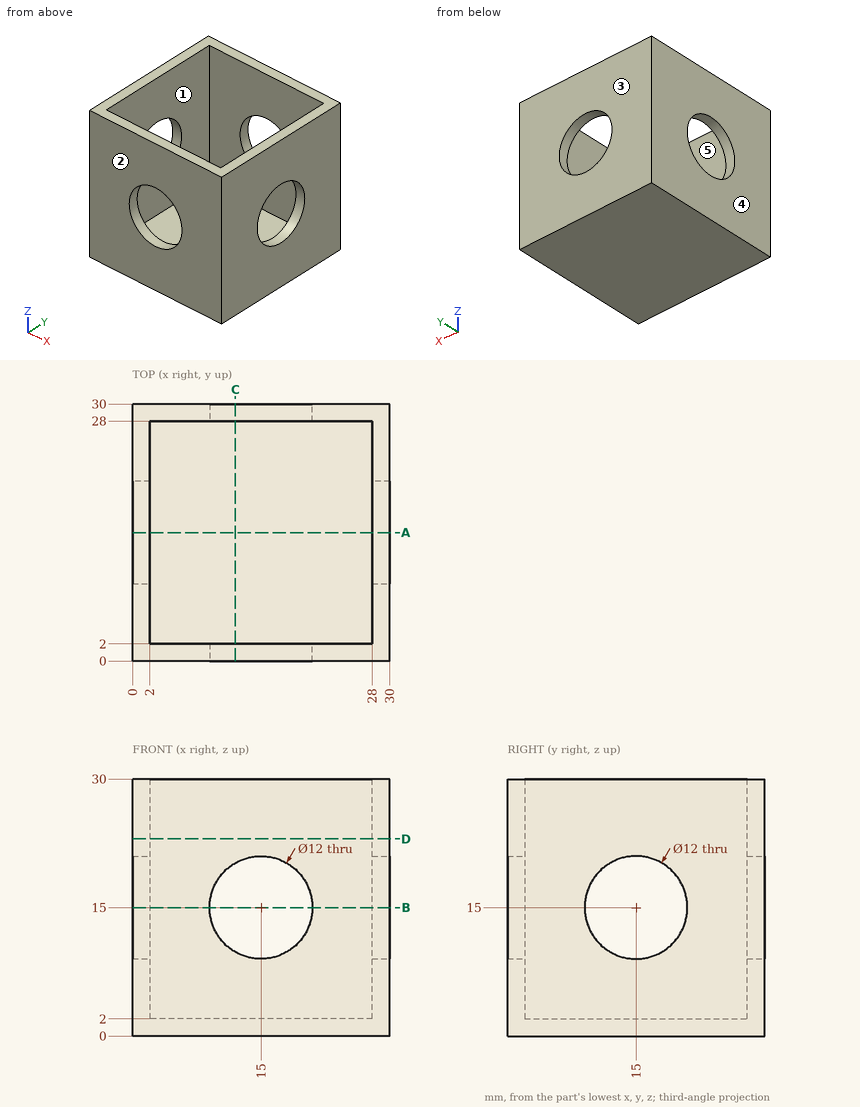
Geometry: see drawing. Coordinates: mm, zero at the bounding-box minimum. A direction names the side the tool comes from. Coordinates: 2 decimals unless noted, no trailing zeros. Order: outer loops, then holes, each group sorted by start corner. A loop starts at its lowest first (then second) coordinate and runs counter-clockwise, first axis right, second up. Notation, with made-up numbers: M 9,21 L 35,21 A18 cw 35,36 Z; hole C 56.5,31 d10. An arc over 180 degrees is marked long. Answer in a Markdown table with one row per item. Add a question column.
Q1. Section query C-C on x = 12. Return the cut outline in (y, z).
Q2. Mould query, pull axis Y, two halves, no side actions, for the marked faces 3, 4 and 5. Classes: released by +Y, released by -Y, zero draft, split by the parting line, or undercut.
Q3. Reachability of the marked faces 1 and 2 from +Z, -Z, +X, -X, +Y, -Y: full face, straight path, thin tool, end or side. Return the list, or none.
Q4. Section query B-B on z = 15. Return the cut outline in (x, y), and give its area (3 significant figures).
Q5. Contact query for a flat-ended pin moving along its axis: P1, Ø9.5, axis at x = 15, z = 15, coming from the +Y side. Output: stop coordinate, or through.
Q6. Section query A-A on y = 15. Return the cut outline in (x, z).
Q7. Section query D-D on z = 23. Return the cut outline in (x, y).
Q8. Line query: L1, parallel to Y at x = 17.5, z = 4.75; L2, parallel to Z at x = 15, y = 28.55. Output: solid intervals per line, ascending.
Completed:
| question | item | result |
|---|---|---|
| 1 | outline | M 0,0 L 30,0 L 30,9.8 L 28,9.8 L 28,2 L 2,2 L 2,9.8 L 0,9.8 Z; M 0,20.2 L 2,20.2 L 2,30 L 0,30 Z; M 28,20.2 L 30,20.2 L 30,30 L 28,30 Z |
| 2 | face 3 | released by +Y |
| 2 | face 4 | zero draft |
| 2 | face 5 | undercut |
| 3 | face 1 | +Z |
| 3 | face 2 | +Z, -Z, +X, -X, -Y |
| 4 | outline | M 0,0 L 9,0 L 9,2 L 2,2 L 2,9 L 0,9 Z; M 0,21 L 2,21 L 2,28 L 9,28 L 9,30 L 0,30 Z; M 21,0 L 30,0 L 30,9 L 28,9 L 28,2 L 21,2 Z; M 21,28 L 28,28 L 28,21 L 30,21 L 30,30 L 21,30 Z |
| 4 | area | 128 mm2 |
| 5 | P1 | passes through |
| 6 | outline | M 0,0 L 30,0 L 30,9 L 28,9 L 28,2 L 2,2 L 2,9 L 0,9 Z; M 0,21 L 2,21 L 2,30 L 0,30 Z; M 28,21 L 30,21 L 30,30 L 28,30 Z |
| 7 | outline | M 0,0 L 30,0 L 30,30 L 0,30 Z; hole M 2,2 L 28,2 L 28,28 L 2,28 Z |
| 8 | L1 | y = 0 to 2, 28 to 30 |
| 8 | L2 | z = 0 to 9, 21 to 30 |
